from build123d import *

# Parameters (mm, degrees)
F0_R     = 10
F1_DEPTH = 5
F2_R     = 4.99999
F3_R     = 3.2
F4_DEPTH = 3


# Not quite as in the source:
# - a fillet or chamfer is up to 0.001 mm smaller than in the source, because OpenCascade refuses the exact size


with BuildPart() as f1:
    # F0 (on Front) → F1 (new body)
    with BuildSketch(Plane.XZ):
        Circle(F0_R)
    extrude(amount=-F1_DEPTH)

    # F2 (radius 5 in the source; OpenCascade refuses exactly that, so slightly less here)
    f2_edges = [f1.edges().sort_by_distance(p)[0] for p in [
        (-10, 5, 0),
    ]]
    fillet(f2_edges, radius=F2_R)

    # F3 (on Front) → F4 (cut)
    with BuildSketch(Plane.XZ):
        Circle(F3_R)
    extrude(amount=-F4_DEPTH, mode=Mode.SUBTRACT)


solid = f1.part
Source: CAD feature listing. Evaluate the final solid. Frame: model axes, mm. A direction names the side the tool comes from. Round coordinates to 2 decimals unless told otherwise and drop trailing zeros. Loops run counter-clockwise (first coordinate to the right, second up) from the corner with the lowest first, then second, coordinate; pieces in that order, holes last. Notation, with made-up numbers: M -10,-10 L 35,-10 A21 ccw 35,26 Z; hole C -20,82 d2. An arc over 180 degrees is marked long. Answer as CSV lines item,"result".
Q1. Contact query for a flat-ended pin moving along its axis: pin 1 (7 mm diameter, centred on x = 0.5, z = 0, fed in from -Y). Output: stop coordinate, or through.
Verdict:
pin 1,"stops at y = 0"
Q2. Line query: line 1 along Z through (x, y) = (0, 0.75); line 2 along Y through (x, z) = (-0.5, -3); line 3 along Z through (x, y) = (0, 1.85). Output: solid intervals per line, ascending.
Verdict:
line 1,"z = -9.94 to -3.2, 3.2 to 9.94"
line 2,"y = 3 to 5"
line 3,"z = -9.65 to -3.2, 3.2 to 9.65"
Q3. Reachability of faces 1 (the face through (-2.539, 1.479, -1.947)), 2 (the face through (-2.4, 0, 2.4)) from +Z, -Z, +X, -X, +Y, -Y: full face, straight path, thin tool, end or side. Return the list, or none.
Verdict:
face 1,"-Y"
face 2,"+Z, -Z, +X, -X, -Y"
Q4. Cut plane C-C (y = 2.2). Return the cut outline in (x, z), plus the area to 3 significant figures.
Verdict:
outline,"C 0,0 d18.98; hole C 0,0 d6.4"
area,"251 mm^2"
Q5. Cut plane D-D (y = 4.65). Return the cut outline in (x, z).
Verdict:
outline,"C 0,0 d13.68"
Q6. Pull-direction query (X, two-part tool) for faces 3 (the face through (0, 5, 0)), 4 (the face through (0, 3, 0)); classes: +X half, -X half, draft (parallel to the pull), parting line (faces both ways), or undercut.
Verdict:
face 3,"draft"
face 4,"undercut"
